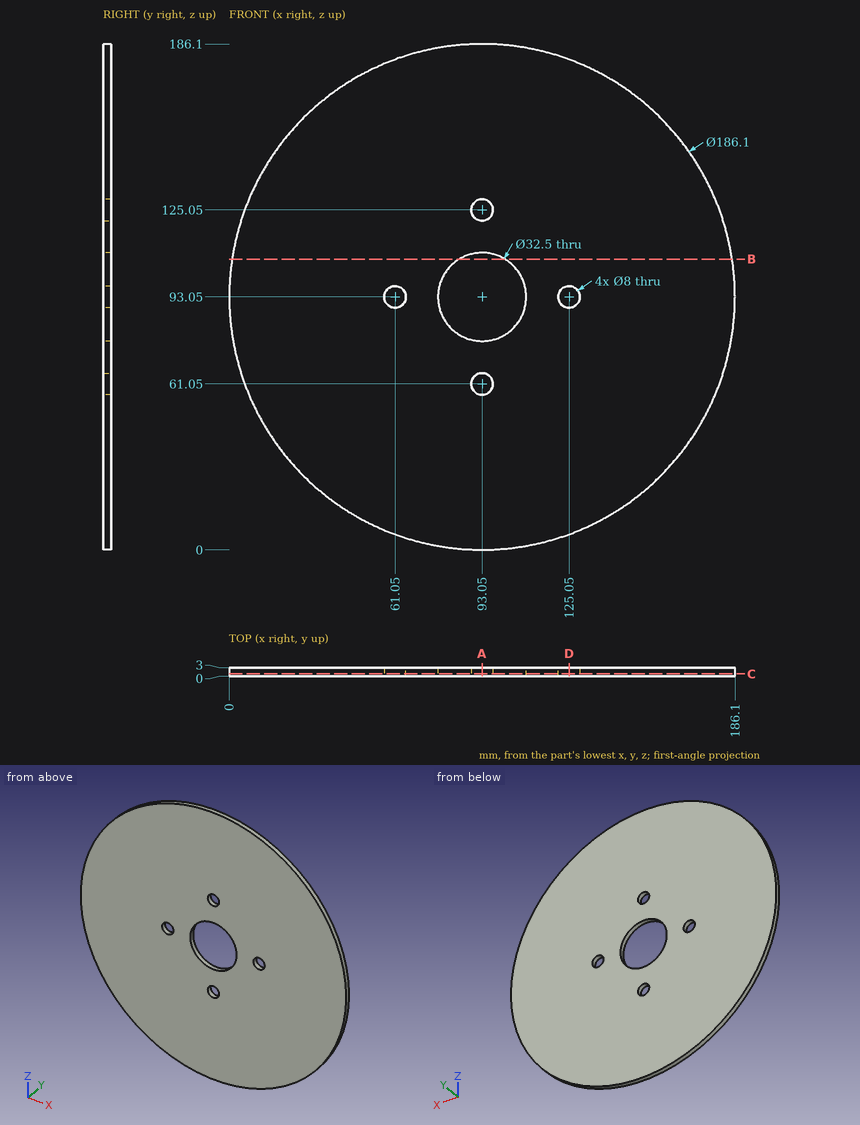
Job drawing, mm, ordinate dimensions from the low corner. One solid piece. Round coordinates to 2 decimals unless told otherwise and drop trailing zeros. Loops run counter-clockwise (first coordinate to the right, second up) from the corner with the lowest first, then second, coordinate; pieces in that order, holes last. Notation, with made-up numbers: (24, 85.5) -> (37, 85.5) arc R34 cw to (37, 115.5) -> close; hole circle Ø9 at (89.5, 59). An arc over 180 degrees is marked (long way). One line per item, written item: value. Start each with the question number.
Q1. Cut at A-A on x = 93.05. List the corners of the cut face in (y, z), plus the area to 3 significant figures.
Q2. Cut at D-D on x = 125.05. List the corners of the cut face in (y, z).
Q3. Cut at B-B on z = 107. List the corners of the cut face in (x, y), plus the area to 3 significant figures.
Q4. Cut at C-C on y = 0.75. List the corners of the cut face in (x, z), plus the area to 3 significant figures.
Q5. Probe line 1 along Z through (x, y) = (93.05, 1.5); line 2 along X through (y, z) = (2.35, 93.5); line 3 along X through (y, z) = (0.35, 60.5). List the from-to ranges inside material, lowest first.
Q6. Drop flat-ended pins along their axis: pin 1 Ø5 at (x, z) = (96, 58.5) entering from +Y; pin 2 Ø19.5 at (x, z) = (93.05, 93.05) entering from +Y. Give the stop position or say it passes through.
Computed:
1. outline: (0, 0) -> (3, 0) -> (3, 57.05) -> (0, 57.05) -> close; (0, 65.05) -> (3, 65.05) -> (3, 76.8) -> (0, 76.8) -> close; (0, 109.3) -> (3, 109.3) -> (3, 121.05) -> (0, 121.05) -> close; (0, 129.05) -> (3, 129.05) -> (3, 186.1) -> (0, 186.1) -> close
1. area: 413 mm²
2. outline: (0, 5.68) -> (3, 5.68) -> (3, 89.05) -> (0, 89.05) -> close; (0, 97.05) -> (3, 97.05) -> (3, 180.42) -> (0, 180.42) -> close
3. outline: (1.05, 0) -> (84.72, 0) -> (84.72, 3) -> (1.05, 3) -> close; (101.38, 0) -> (185.05, 0) -> (185.05, 3) -> (101.38, 3) -> close
3. area: 502 mm²
4. outline: circle Ø186.1 at (93.05, 93.05); hole circle Ø8 at (61.05, 93.05); hole circle Ø32.5 at (93.05, 93.05); hole circle Ø8 at (93.05, 61.05); hole circle Ø8 at (93.05, 125.05); hole circle Ø8 at (125.05, 93.05)
4. area: 26,200 mm²
5. line 1: 0 to 57.05, 65.05 to 76.8, 109.3 to 121.05, 129.05 to 186.1
5. line 2: 0 to 57.08, 65.02 to 76.81, 109.29 to 121.08, 129.02 to 186.1
5. line 3: 5.88 to 89.09, 97.01 to 180.22
6. pin 1: y = 3
6. pin 2: through
